Can you work these out from the model? Positions are in its coordinate system, mm. Give positions to 0.01 mm unless a question says otherwise; leave off trailing zeros. Loops run counter-clockwise (first coordinate to the right, second up) from the corner with the lowest first, then second, coordinate; pieces in that order, holes last. Notation, with made-up numbers: M 42.5,-0.75 L 76.5,-0.75 A13 ccw 76.5,7.25 Z; hole C -31.75,-33 d5. An arc over 180 degrees is marked long. Use CSV: the item, a comma, the result in double quotes.
from build123d import *

# Parameters (mm, degrees)
F2_R     = 0.5
F3_SIZE2 = 0.5
F3_SIZE  = 2


with BuildPart() as f1:
    # F0 (on Front) → F1 (revolve)
    with BuildSketch(Plane.XZ):
        with BuildLine():
            Line((0, 18), (0, 0))
            Line((0, 0), (4.525, 0))
            Line((4.525, 0), (4.525, 11.681882))
            ThreePointArc((4.525, 11.681882), (4.389009, 12.782892), (3.989211, 13.817724))
            Line((3.989211, 13.817724), (1.75, 18))
            Line((1.75, 18), (0, 18))
        make_face()
    revolve(axis=Axis((0, 0, -7.393045), (0, 0, -1)))

    # F2
    f2_edges = [f1.edges().sort_by_distance(p)[0] for p in [
        (-1.75, 0, 18),
    ]]
    fillet(f2_edges, radius=F2_R)

    # F3
    f3_edges = [f1.edges().sort_by_distance(p)[0] for p in [
        (-4.525, 0, 0),
    ]]
    chamfer(f3_edges, length=F3_SIZE, length2=F3_SIZE2)


solid = f1.part
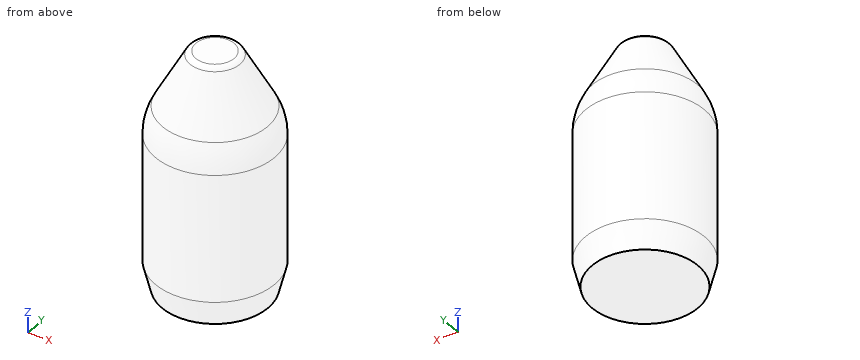
Q1. Please list where these lines run through material, in increasing order: L1, parallel to X at y = -2.5, z = 2.5; L2, parallel to Y at x = 2, z = 6.25. Write a range as from..to.
Model answer:
L1,"-3.77..3.77"
L2,"-4.06..4.06"
Q2. I want a section at A-A, the plane z = 2.75. Please give me the cut outline in (x, y) (3 decimals), then the cut area to 3 significant figures.
Model answer:
outline,"C 0,0 d9.05"
area,"64.3 mm2"
Q3. I'm going to push flat-ended pins straight in: P1, Ø2, axis at y = 3, z = 13, coming from the +X side; P2, Ø2, axis at y = -2, z = 10.5, coming from the -X side; P3, Ø2, axis at y = 1.5, z = 8.5, coming from the +X side. Where does each tip first touch, or does it pass through?
Model answer:
P1,"x = 3.91"
P2,"x = -4.41"
P3,"x = 4.5"
Q4. I want a section at B-B, the plane z = 14.75. Please give me the cut outline in (x, y), then the cut area to 3 significant figures.
Model answer:
outline,"C 0,0 d6.98"
area,"38.3 mm2"
